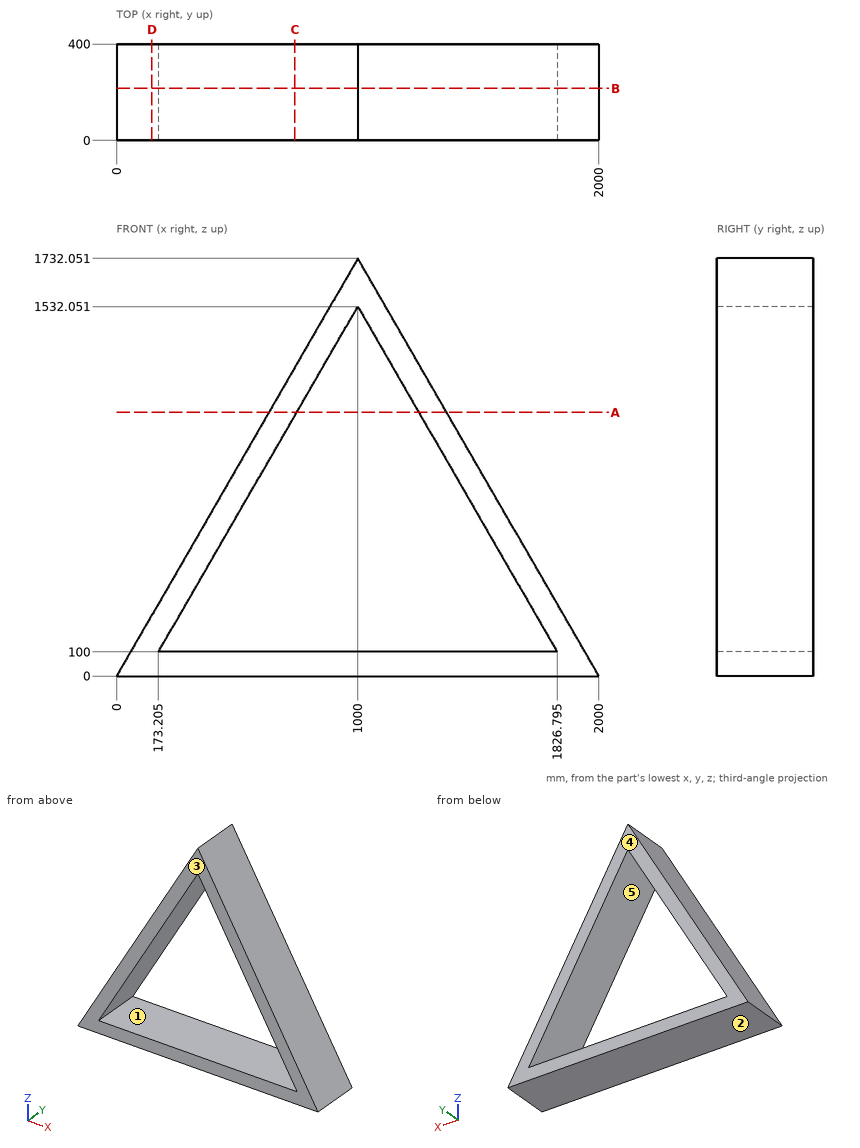
For this review, use the dimensioned drawing (mm, ordinates from the lowest corner) and the shaded views. A direction names the side the tool comes from. Give positions to 0.01 mm unless a question says otherwise; leave off trailing zeros. Write each loop counter-clockwise with the first axis right and the second up, starting at its lowest first coordinate (ties: lowest second). Pieces come first, ordered by that corner, then holes.
(1) Consider section A-A, the plane z = 1093. Give the boundary of the cut face in (x, y).
(2) Tool access review of the marked faces 4 and 5: name each direction out of +Z, -Z, +X, -X, +Y, -Y from which nothing blocks a thin tool from reaching the whole face with its end or side.
(3) Consider section D-D, the plane x = 145.5. Give the boundary of the cut face in (y, z).
(4) Consider section B-B, the plane y = 215.5. Give the boundary of the cut face in (x, z) (1 decimal), and give its area (3 significant figures).
(5) The part is to be moulded in two halves that separate along Z. For the marked faces 1, 2 and 3, say which applies: released by +Z, released by -Z, zero draft, split by the parting line, or undercut.
(6) For P1, Ø12, axis at x = 1766, y = 284.5, coming from the +Z side; P2, Ø1.5, axis at y = 337.5, z = 218.5, coming from the +X side, all flat-tipped, find the tip position at first contact; note any pin that passes through.
(7) To check wall thickness, follow L1, parallel to Z at x = 1049, y = 43.5; L2, parallel to X at y = 109.5, z = 1213.5 (1 decimal); L3, parallel to X at y = 132, z = 568 (1 decimal). State the ranges of each line that lie inside material, in increasing order.
(8) Consider section C-C, the plane x = 739. Give the boundary of the cut face in (y, z), and give its area (3 significant figures).
Returned:
1. outline: (631.04, 0) - (746.51, 0) - (746.51, 400) - (631.04, 400) - close; (1253.49, 0) - (1368.96, 0) - (1368.96, 400) - (1253.49, 400) - close
2. face 4: +Z, -Z, +X, -X, +Y
2. face 5: +Y, -Y
3. outline: (0, 0) - (400, 0) - (400, 252.01) - (0, 252.01) - close
4. outline: (0, 0) - (2000, 0) - (1000, 1732.1) - close; hole (173.2, 100) - (1826.8, 100) - (1000, 1532.1) - close
4. area: 548,000 mm2
5. face 1: undercut
5. face 2: released by -Z
5. face 3: zero draft
6. P1: stops at z = 415.69
6. P2: stops at x = 1874.28
7. L1: z = 0 to 100, 1447.18 to 1647.18
7. L2: x = 700.6 to 816.1, 1183.9 to 1299.4
7. L3: x = 327.9 to 443.4, 1556.6 to 1672.1
8. outline: (0, 0) - (400, 0) - (400, 100) - (0, 100) - close; (0, 1079.99) - (400, 1079.99) - (400, 1279.99) - (0, 1279.99) - close
8. area: 120,000 mm2
